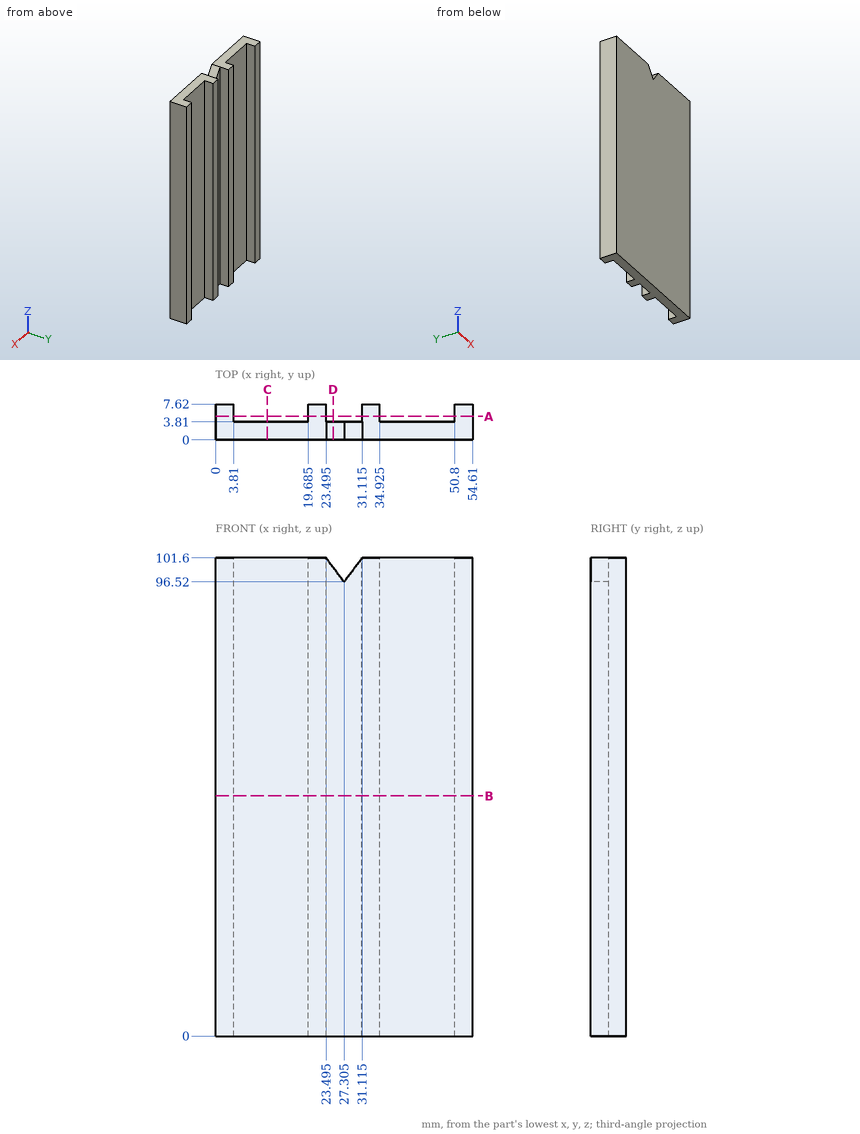
Here's the drawing with two shaded views (mm, measured from the low corner). I have some questions. Coordinates: 2 decimals unless noted, no trailing zeros. Loops run counter-clockwise (first coordinate to the right, second up) from the corner with the lowest first, then second, coordinate; pieces in that order, holes last. Notation, with made-up numbers: M 80.25,-28.5 L 104.25,-28.5 A20 cw 104.25,-17.5 Z; hole C -9.75,89 d5. An arc over 180 degrees is marked long. Answer as CSV lines item,"result". Start each with the question number.
1. Suppose I cut it at A-A, the plane y = 5. List the corners of the cut face in (x, z) for me (3 decimals), plus the area to 3 significant figures.
2. Suppose I cut it at D-D, the plane x = 25. List the corners of the cut face in (y, z) for me, plus the area to 3 significant figures.
3. Suppose I cut it at C-C, the plane x = 11. List the corners of the cut face in (y, z) for me.
4. For pin 1 Ø4 at (y, z) = (6, 30) entering from -X; pin 2 Ø1.5 at (x, y) = (6, 6) entering from +Z; pin 3 Ø4 at (x, z) = (26, 65.5) entering from +Y, each with a flat end and sliding along its axis, tell me the tip position at first contact or that it passes through.
5. If I drill on probe 1 along X at (y, z) = (5, 30) (3 decimals); probe 2 along Y at (x, z) = (37, 89); probe 3 along Z at (x, y) = (25, 0.5), over which ranges is the centre line in solid material (lowest first)? Write a range as [from, to].
6. Suppose I cut it at B-B, the plane z = 51. List the corners of the cut face in (x, y) for me (3 decimals), plus the area to 3 significant figures.
Output:
1,outline,"M 0,0 L 3.81,0 L 3.81,101.6 L 0,101.6 Z; M 19.685,0 L 23.495,0 L 23.495,101.6 L 19.685,101.6 Z; M 31.115,0 L 34.925,0 L 34.925,101.6 L 31.115,101.6 Z; M 50.8,0 L 54.61,0 L 54.61,101.6 L 50.8,101.6 Z"
1,area,"1,550 mm^2"
2,outline,"M 0,0 L 3.81,0 L 3.81,99.59 L 0,99.59 Z"
2,area,"379 mm^2"
3,outline,"M 0,0 L 3.81,0 L 3.81,101.6 L 0,101.6 Z"
4,pin 1,"stops at x = 0"
4,pin 2,"passes through"
4,pin 3,"stops at y = 3.81"
5,probe 1,"x = [0, 3.81], [19.685, 23.495], [31.115, 34.925], [50.8, 54.61]"
5,probe 2,"y = [0, 3.81]"
5,probe 3,"z = [0, 99.59]"
6,outline,"M 0,0 L 54.61,0 L 54.61,7.62 L 50.8,7.62 L 50.8,3.81 L 34.925,3.81 L 34.925,7.62 L 31.115,7.62 L 31.115,3.81 L 23.495,3.81 L 23.495,7.62 L 19.685,7.62 L 19.685,3.81 L 3.81,3.81 L 3.81,7.62 L 0,7.62 Z"
6,area,"266 mm^2"
